Input: dimensioned drawing with shaded views. Units: mm. Origin: part minimum x, y, z. Round coordinates to 2 decimals unless told otherwise and drop trailing zeros. Loops run counter-clockwise (first coordinate to the right, second up) from the corner with the lowest first, then second, coordinate; pieces in that order, holes last. Notation, with made-up numbers: (17.25, 57) -> (34.25, 57) arc R24 ccw to (34.25, 87) -> close; hole circle Ø9 at (-16, -15.5). An arc over 180 degrees is marked (long way). Answer as a JSON object with one key per item and string values.
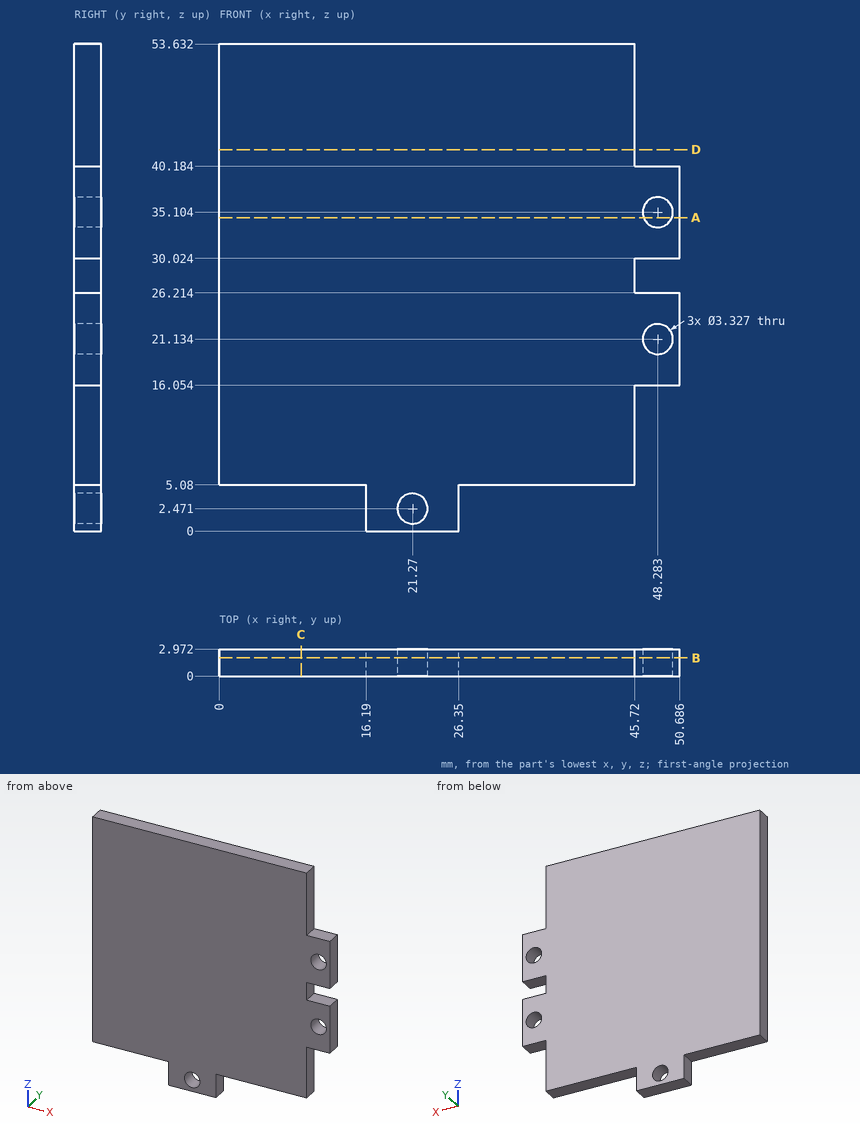
1) Ray query, probe 1 along Z at (x, y) = (48.5, 2) (1 decimal); probe 2 along X at (y, z) = (1.9, 35) (1 decimal); probe 3 along Z at (x, y) = (14.5, 2.3). Return the intervals inside material, ascending.
Output:
{"probe 1": "z = 16.1 to 19.5, 22.8 to 26.2, 30 to 33.5, 36.8 to 40.2", "probe 2": "x = 0 to 46.6, 49.9 to 50.7", "probe 3": "z = 5.08 to 53.63"}
2) Contact query for flat-ended pins moving along their axis: P1, Ø0.9, axis at y = 2, z = 12.5, coming from the +X side; P2, Ø0.9, axis at x = 47.5, y = 1, coming from the +Z side; P3, Ø1.5, axis at y = 1.5, z = 2.5, coming from the -X side. Output: stop coordinate, or through.
Output:
{"P1": "stops at x = 45.72", "P2": "stops at z = 40.18", "P3": "stops at x = 16.19"}
3) Section B-B, the plane y = 2. Count the separate pieces of the cut face and the enclosed holes in it, plus the area to 3 significant figures.
Output:
{"separate pieces": "1", "enclosed holes": "3", "area": "2,350 mm^2"}
4) Section A-A, the plane z = 34.5. Output: boundary loops of the cut face in (x, y) (1 decimal).
Output:
{"outline": "(0, 0) -> (46.7, 0) -> (46.7, 3) -> (0, 3) -> close; (49.8, 0) -> (50.7, 0) -> (50.7, 3) -> (49.8, 3) -> close"}
5) Section C-C, the plane x = 9. Output: boundary loops of the cut face in (y, z).
Output:
{"outline": "(0, 5.08) -> (2.97, 5.08) -> (2.97, 53.63) -> (0, 53.63) -> close"}
6) Section D-D, the plane z = 42. Output: boundary loops of the cut face in (x, y), plus the area to 3 significant figures.
Output:
{"outline": "(0, 0) -> (45.72, 0) -> (45.72, 2.97) -> (0, 2.97) -> close", "area": "136 mm^2"}
